CAD build for the part. Positions are in the model's coordinates, mm. Face numbers are marked on the shaded views. A direction names the side the tool comes from. Round coordinates to 2 decimals unless told otherwise and drop trailing zeros. Loops run counter-clockwise (first coordinate to the right, second up) from the corner with the lowest first, then second, coordinate; pieces in that order, holes last.
from build123d import *

# Parameters (mm, degrees)
SKETCH_1_W                         = 30
SKETCH_1_H                         = 20
SM_BASE_FLANGE_1_DEPTH             = 4
SM_EDGE_FLANGE_1_STRIP_W           = 18
SM_EDGE_FLANGE_1_STRIP_H           = 4
SM_EDGE_FLANGE_1_STRIP_CUT_DEPTH   = 20
SM_EDGE_FLANGE_1_STRIP_2_W         = 18
SM_EDGE_FLANGE_1_STRIP_2_H         = 4
SM_EDGE_FLANGE_1_STRIP_CUT_2_DEPTH = 20
SM_EDGE_FLANGE_1_DEPTH             = 20
SM_EDGE_FLANGE_1_BEND_DEPTH        = 20
FILLET_1_R                         = 3
SKETCH_12_R                        = 3
CUT_EXTRUDE_1_DEPTH                = 10
SKETCH_13_R                        = 3
CUT_EXTRUDE_2_DEPTH                = 64.592452382


# Sheet-metal steps are written as plain solids
with BuildPart() as part:
    # Sketch 1 → 基体-法兰1 (new body)
    with BuildSketch(Plane.XY):
        Rectangle(SKETCH_1_W, SKETCH_1_H)
    extrude(amount=-SM_BASE_FLANGE_1_DEPTH)

    # 边线-法兰1 strip (across the edge) → 边线-法兰1 strip cut (cut)
    with BuildSketch(Plane(origin=(-15, 10, 0), x_dir=(1, 0, 0), z_dir=(0, -1, 0))):
        with Locations((-8, -2)):
            Rectangle(SM_EDGE_FLANGE_1_STRIP_W, SM_EDGE_FLANGE_1_STRIP_H)
    extrude(amount=SM_EDGE_FLANGE_1_STRIP_CUT_DEPTH, mode=Mode.SUBTRACT)

    # 边线-法兰1 strip 2 (across the edge) → 边线-法兰1 strip cut 2 (cut)
    with BuildSketch(Plane(origin=(15, -10, 0), x_dir=(-1, 0, 0), z_dir=(0, 1, 0))):
        with Locations((-8, -2)):
            Rectangle(SM_EDGE_FLANGE_1_STRIP_2_W, SM_EDGE_FLANGE_1_STRIP_2_H)
    extrude(amount=SM_EDGE_FLANGE_1_STRIP_CUT_2_DEPTH, mode=Mode.SUBTRACT)

    # 边线-法兰1 section (across the edge) → 边线-法兰1 (add)
    with BuildSketch(Plane(origin=(-15, 10, 0), x_dir=(1, 0, 0), z_dir=(0, -1, 0))):
        with BuildLine():
            Line((-4, 1), (-4, 50))
            Line((-4, 50), (0, 50))
            Line((0, 50), (0, 1))
            ThreePointArc((0, 1), (0.292893219, 0.292893219), (1, 0))
            Line((1, 0), (1, -4))
            ThreePointArc((1, -4), (-2.535533906, -2.535533906), (-4, 1))
        make_face()
    extrude(amount=SM_EDGE_FLANGE_1_DEPTH)

    # 边线-法兰1 section 2 (across the edge) → 边线-法兰1 bend (add)
    with BuildSketch(Plane(origin=(15, -10, 0), x_dir=(-1, 0, 0), z_dir=(0, 1, 0))):
        with BuildLine():
            Line((-4, 1), (-4, 50))
            Line((-4, 50), (0, 50))
            Line((0, 50), (0, 1))
            ThreePointArc((0, 1), (0.292893219, 0.292893219), (1, 0))
            Line((1, 0), (1, -4))
            ThreePointArc((1, -4), (-2.535533906, -2.535533906), (-4, 1))
        make_face()
    extrude(amount=SM_EDGE_FLANGE_1_BEND_DEPTH)

    # 圆角1
    fillet_1_edges = [part.edges().sort_by_distance(p)[0] for p in [
        (-17, 10, 50),
        (-17, -10, 50),
        (17, -10, 50),
        (17, 10, 50),
    ]]
    fillet(fillet_1_edges, radius=FILLET_1_R)

    # 草图12 → 切除-拉伸1 (cut)
    with BuildSketch(Plane.XY):
        Circle(SKETCH_12_R)
    extrude(amount=-CUT_EXTRUDE_1_DEPTH, mode=Mode.SUBTRACT)

    # 草图13 → 切除-拉伸2 (cut, through all)
    with BuildSketch(Plane.ZY.offset(19)):
        with Locations((42, 0)):
            Circle(SKETCH_13_R)
    extrude(amount=-CUT_EXTRUDE_2_DEPTH, mode=Mode.SUBTRACT)


solid = part.part
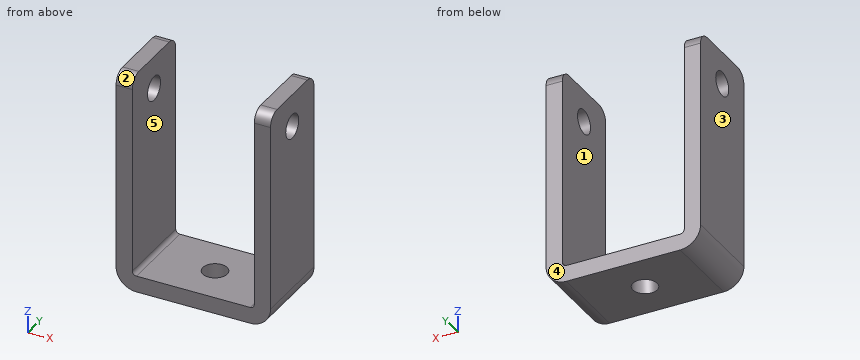
Item 1: Cut at A-A (z = 37.5). List the corners of the cut face in (x, y).
Verdict:
outline: (-19, -10) - (-15, -10) - (-15, 10) - (-19, 10) - close; (15, -10) - (19, -10) - (19, 10) - (15, 10) - close
Item 2: Cut at C-C (y = 0). List the corners of the cut face in (x, z), plus the area to 3 significant figures.
Verdict:
outline: (-19, 1) arc R5 ccw to (-14, -4) - (-3, -4) - (-3, 0) - (-14, 0) arc R1 cw to (-15, 1) - (-15, 39) - (-19, 39) - close; (-19, 45) - (-15, 45) - (-15, 50) - (-19, 50) - close; (3, -4) - (14, -4) arc R5 ccw to (19, 1) - (19, 39) - (15, 39) - (15, 1) arc R1 cw to (14, 0) - (3, 0) - close; (15, 45) - (19, 45) - (19, 50) - (15, 50) - close
area: 470 mm2
Item 3: Flat gauge pin, fed straight in: P1, Ø6, axis at x = 0.5, y = -3.5, coming from the +Z side. Where does the tip first touch, or does it go through?
Verdict:
P1: stops at z = 0
Item 4: Cut at B-B (x = 0). List the corners of the cut face in (y, z).
Verdict:
outline: (-10, -4) - (-3, -4) - (-3, 0) - (-10, 0) - close; (3, -4) - (10, -4) - (10, 0) - (3, 0) - close
Item 5: Cut at D-D (x = 17). List the corners of the cut face in (y, z).
Verdict:
outline: (-10, -3) - (10, -3) - (10, 47) arc R3 ccw to (7, 50) - (-7, 50) arc R3 ccw to (-10, 47) - close; hole circle Ø6 at (0, 42)
Item 6: Wall check: L1, parallel to X at y = 8.25, z = 28; L2, parallel to Y at x = 0, z = -1.8; L3, parallel to Z at x = -4.5, y = 2.5. Give the ranges that are in metal, low to high.
Verdict:
L1: x = -19 to -15, 15 to 19
L2: y = -10 to -3, 3 to 10
L3: z = -4 to 0
Item 7: 3-axis set-ups, long thin cutter, end or side, ignore diameter. For the marked faces 1 and 2: which of +Z, -Z, +X, -X, +Y, -Y reach the whole face in a straight line?
Verdict:
face 1: +Z, +Y, -Y
face 2: +Z, +X, -X, -Y
Item 8: Mould opens along X. For the marked faces 3, 4 and 5 say: released by +X, released by -X, zero draft, split by the parting line, or undercut.
Verdict:
face 3: released by -X
face 4: zero draft
face 5: undercut
